Design review of the part built by this model. Coordinates are the model's own, in mm. Face numbers are marked on the shaded views. A direction names the side the tool comes from. Coordinates: 2 decimals unless noted, no trailing zeros. Write each loop counter-clockwise with the first axis right and the second up, starting at its lowest first coordinate (ties: lowest second). Pieces come first, ordered by that corner, then holes.
Q1. Take a section at A-A (x = 0). Give the boundary of the cut face in (y, z).
Q2. For probe 1 along Y at (x, z) = (-1.3, -1.1); probe 2 along X at (y, z) = (2.8, 0), list the stretches that pass through material, from the lowest coordinate up.
Q3. Insertion check: pin 1 (0.6 mm diameter, centred on x = 1.5, y = 9, fed in from -Z); pin 2 (0.8 mm diameter, centred on x = 1.5, y = 1.5, fed in from +Z); pin 3 (1 mm diameter, centred on y = 5, z = -1, fed in from -X). Each pin has a flat end and moves straight along its axis. Give the tip position at first contact, or say it passes through.
Q4. Take a section at D-D (z = 1.65). Give the boundary of the cut face in (x, y), and give its area (3 significant figures).
Q5. Mouldability with a two-part tool opening along Y and no side actions: class the marked faces 3, 4 and 5 as pulls with the +Y half, pulls with the -Y half, needs draft (parallel to the pull), parting line crosses it, or undercut.
Q6. Machinability: for the marked faces 1 and 2, which of the approach directions +Z, -Z, +X, -X, +Y, -Y give a long, thin tool a straight path to every point of the face, cutting with its end or side? Answer none if there is none.
Q7. Take a section at B-B (z = -0.65). Give the boundary of the cut face in (x, y), and give its area (3 significant figures).
Q8. Take a section at C-C (y = 1). Give the boundary of the cut face in (x, z), and give its area (3 significant figures).
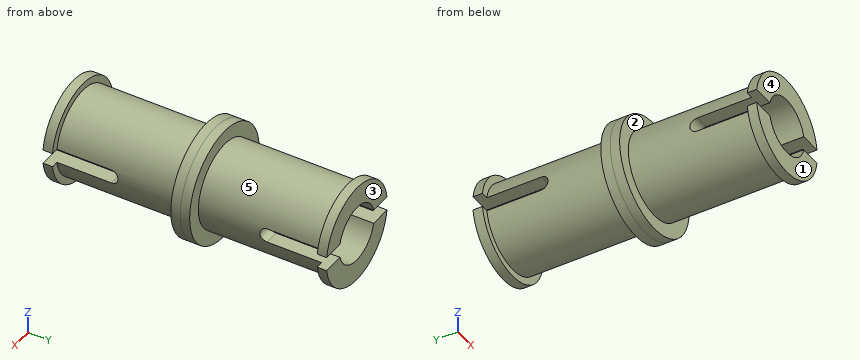
```python
from build123d import *

# Parameters (mm, degrees)
SKETCH1_R               = 1.5
SKETCH1_R_2             = 1
BOSS_EXTRUDE1_DEPTH     = 5
SKETCH2_R               = 2
SKETCH2_R_2             = 1
BOSS_EXTRUDE2_DEPTH     = 0.333333333
SKETCH3_R               = 1.75
SKETCH3_R_2             = 1
BOSS_EXTRUDE4_DEPTH     = 0.333333333
SKETCH4_R               = 0.25
SKETCH4_W               = 0.5
SKETCH4_H               = 2.25
CUT_EXTRUDE1_DEPTH      = 3
CUT_EXTRUDE1_DEPTH_BACK = 3


with BuildPart() as part:
    # Sketch1 → Boss-Extrude1 (new body)
    with BuildSketch(Plane(origin=(0, 0, 0), x_dir=(1, 0, 0), z_dir=(0, 1, 0))):
        Circle(SKETCH1_R)
        Circle(SKETCH1_R_2, mode=Mode.SUBTRACT)
    extrude(amount=BOSS_EXTRUDE1_DEPTH)

    # Sketch2 → Boss-Extrude2 (add)
    with BuildSketch(Plane(origin=(0, 5, 0), x_dir=(1, 0, 0), z_dir=(0, 1, 0))):
        Circle(SKETCH2_R)
        Circle(SKETCH2_R_2, mode=Mode.SUBTRACT)
    extrude(amount=-BOSS_EXTRUDE2_DEPTH)

    # Sketch3 → Boss-Extrude4 (add)
    with BuildSketch(Plane(origin=(0, 0, 0), x_dir=(-1, 0, 0), z_dir=(0, -1, 0))):
        Circle(SKETCH3_R)
        Circle(SKETCH3_R_2, mode=Mode.SUBTRACT)
    extrude(amount=-BOSS_EXTRUDE4_DEPTH)

    # Sketch4 → Cut-Extrude1 (cut, two sides)
    with BuildSketch(Plane(origin=(0, 0, 0), x_dir=(0, 0, -1), z_dir=(1, 0, 0))) as cut_extrude1_sk:
        with Locations((0, 2.25)):
            Circle(SKETCH4_R)
        with Locations((0, 1.125)):
            Rectangle(SKETCH4_W, SKETCH4_H)
    extrude(amount=CUT_EXTRUDE1_DEPTH, mode=Mode.SUBTRACT)
    extrude(cut_extrude1_sk.sketch, amount=-CUT_EXTRUDE1_DEPTH_BACK, mode=Mode.SUBTRACT)

    # Mirror1: part across plane


with BuildPart() as part_1:
    add(part.part)
    add(part.part.mirror(Plane.ZX.offset(5)))


solid = part_1.part
```
Response:
1. outline: (0, -1.75) - (0.33, -1.75) - (0.33, -1.5) - (4.67, -1.5) - (4.67, -2) - (5.33, -2) - (5.33, -1.5) - (9.67, -1.5) - (9.67, -1.75) - (10, -1.75) - (10, -1) - (0, -1) - close; (0, 1) - (10, 1) - (10, 1.75) - (9.67, 1.75) - (9.67, 1.5) - (5.33, 1.5) - (5.33, 2) - (4.67, 2) - (4.67, 1.5) - (0.33, 1.5) - (0.33, 1.75) - (0, 1.75) - close
2. probe 1: y = 0 to 0.33, 4.67 to 5.33, 9.67 to 10
2. probe 2: x = -1.5 to -1, 1 to 1.5
3. pin 1: stops at z = -0.9
3. pin 2: stops at z = 1.02
3. pin 3: stops at x = -1.94
4. outline: (-1.13, 4.67) - (1.13, 4.67) - (1.13, 5.33) - (-1.13, 5.33) - close; (-0.58, 0) - (0.58, 0) - (0.58, 0.33) - (-0.58, 0.33) - close; (-0.58, 9.67) - (0.58, 9.67) - (0.58, 10) - (-0.58, 10) - close
4. area: 2.28 mm2
5. face 3: pulls with the +Y half
5. face 4: pulls with the -Y half
5. face 5: undercut
6. face 1: +Z, -Z, +X, -X, -Y
6. face 2: none
7. outline: (-1.89, 4.67) - (-1.35, 4.67) - (-1.35, 0.33) - (-1.62, 0.33) - (-1.62, 0) - (-0.76, 0) - (-0.76, 10) - (-1.62, 10) - (-1.62, 9.67) - (-1.35, 9.67) - (-1.35, 5.33) - (-1.89, 5.33) - close; (0.76, 0) - (1.62, 0) - (1.62, 0.33) - (1.35, 0.33) - (1.35, 4.67) - (1.89, 4.67) - (1.89, 5.33) - (1.35, 5.33) - (1.35, 9.67) - (1.62, 9.67) - (1.62, 10) - (0.76, 10) - close
7. area: 12.9 mm2
8. outline: (-1.48, -0.25) arc R1.5 ccw to (1.48, -0.25) - (0.97, -0.25) arc R1 cw to (-0.97, -0.25) - close; (-1.48, 0.25) - (-0.97, 0.25) arc R1 cw to (0.97, 0.25) - (1.48, 0.25) arc R1.5 ccw to start
8. area: 3.42 mm2
